from build123d import *

# Parameters (mm, degrees)
ESQUISSE2_R          = 3.75
BOSS_EXTRU_1_DEPTH   = 4
BOSS_EXTRU_1_2_DEPTH = 4
BOSS_EXTRU_1_3_DEPTH = 4
BOSS_EXTRU_1_4_DEPTH = 4
ESQUISSE3_R          = 17
ESQUISSE3_R_2        = 14.5
BOSS_EXTRU_2_DEPTH   = 4
CONG_1_R             = 2
CONG_2_R             = 2
PER_AGE1_D           = 4
PER_AGE1_DEPTH       = 93.98


with BuildPart() as part:
    # Esquisse2 → Boss.-Extru.1 (new body)
    with BuildSketch(Plane.XY):
        with Locations((-12, 12)):
            Circle(ESQUISSE2_R)
    extrude(amount=BOSS_EXTRU_1_DEPTH)



with BuildPart() as body_2:
    # Esquisse2 → Boss.-Extru.1 2 (new body)
    with BuildSketch(Plane.XY):
        with Locations((12, 12)):
            Circle(ESQUISSE2_R)
    extrude(amount=BOSS_EXTRU_1_2_DEPTH)


with BuildPart() as body_3:
    # Esquisse2 → Boss.-Extru.1 3 (new body)
    with BuildSketch(Plane.XY):
        with Locations((-12, -12)):
            Circle(ESQUISSE2_R)
    extrude(amount=BOSS_EXTRU_1_3_DEPTH)


with BuildPart() as body_4:
    # Esquisse2 → Boss.-Extru.1 4 (new body)
    with BuildSketch(Plane.XY):
        with Locations((12, -12)):
            Circle(ESQUISSE2_R)
    extrude(amount=BOSS_EXTRU_1_4_DEPTH)


with BuildPart() as part_1:
    add(part.part)

    add(body_2.part)  # Boss.-Extru.2 merges body 2

    add(body_3.part)  # Boss.-Extru.2 merges body 3

    add(body_4.part)  # Boss.-Extru.2 merges body 4
    # Esquisse3 → Boss.-Extru.2 (add)
    with BuildSketch(Plane.XY):
        Circle(ESQUISSE3_R)
        Circle(ESQUISSE3_R_2, mode=Mode.SUBTRACT)
    extrude(amount=BOSS_EXTRU_2_DEPTH)

    # Congé1
    cong_1_edges = [part_1.edges().sort_by_distance(p)[0] for p in [
        (-14.365513596, 9.09021557, 2),
        (-9.09021557, 14.365513596, 2),
        (14.365513596, 9.09021557, 2),
        (9.09021557, 14.365513596, 2),
        (-14.365513596, -9.09021557, 2),
        (-9.09021557, -14.365513596, 2),
        (9.09021557, -14.365513596, 2),
        (14.365513596, -9.09021557, 2),
    ]]
    fillet(cong_1_edges, radius=CONG_1_R)

    # Congé2
    cong_2_edges = [part_1.edges().sort_by_distance(p)[0] for p in [
        (-11.92370292, 8.250776246, 2),
        (-8.250776246, 11.92370292, 2),
        (8.250776246, 11.92370292, 2),
        (11.92370292, 8.250776246, 2),
        (-11.92370292, -8.250776246, 2),
        (-8.250776246, -11.92370292, 2),
        (8.250776246, -11.92370292, 2),
        (11.92370292, -8.250776246, 2),
    ]]
    fillet(cong_2_edges, radius=CONG_2_R)

    # Perçage1
    with Locations(Plane(origin=(0, 0, 0), x_dir=(-1, 0, 0), z_dir=(0, 0, -1))):
        with Locations((-12, 12), (12, 12), (12, -12), (-12, -12)):
            Hole(PER_AGE1_D / 2, depth=PER_AGE1_DEPTH)


solid = part_1.part
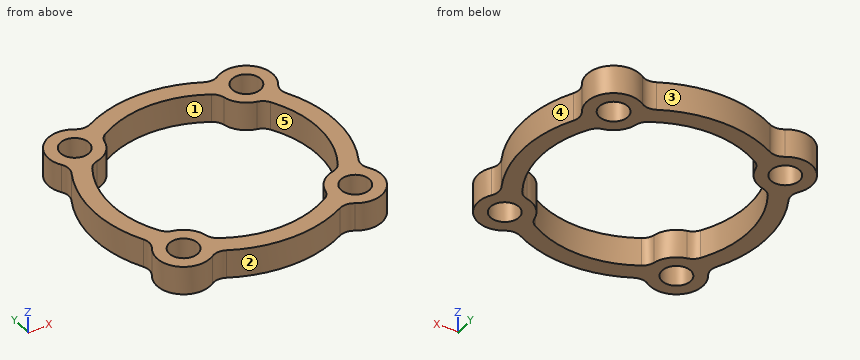
Design review of the part built by this model. Coordinates are the model's own, in mm. Face numbers are marked on the shaded views. A direction names the side the tool comes from. Give positions to 0.01 mm unless a question says otherwise; leave off trailing zeros. Loops run counter-clockwise (first coordinate to the right, second up) from the corner with the lowest first, then second, coordinate; pieces in that order, holes last. Notation, with made-up numbers: M 5.5,-19.5 L 52.5,-19.5 A27 cw 52.5,-3.5 Z; hole C 0.5,35 d10. An arc over 180 degrees is marked long. Answer as a JSON object with one key per item and string values.
Item 1: We need section B-B (z = 0.55). Count the separate pieces of the cut face and the enclosed holes in it, and give its area (3 significant figures).
Output values:
{"separate pieces": "1", "enclosed holes": "5", "area": "310 mm2"}
Item 2: Wall thickness on line 1 along Y through (x, z) = (-12, 2.95); line 2 along X through (y, z) = (-11, 0.95); line 3 along X through (y, z) = (-13, 3.45): over which ranges is each line inside the solid? List them lowest first.
Output values:
{"line 1": "y = -15.75 to -14, -10 to -7.95, 7.95 to 10, 14 to 15.75", "line 2": "x = -15.61 to -13.73, -10.27 to -8.39, 8.39 to 10.27, 13.73 to 15.61", "line 3": "x = -15.61 to -13.73, -10.27 to -6.42, 6.42 to 10.27, 13.73 to 15.61"}
Item 3: Mouldability with a two-part tool opening along Y and no side actions: class the marked faces 1, 2 and 3 as pulls with the +Y half, pulls with the -Y half, needs draft (parallel to the pull), parting line crosses it, or undercut.
Output values:
{"face 1": "undercut", "face 2": "pulls with the -Y half", "face 3": "pulls with the +Y half"}
Item 4: For P1, Ø1, axis at x = -0.5, z = 0.5, coming from the +Y side; P2, Ø8, axis at x = 4, y = 7.5, coming from the +Z side; P3, Ø2, axis at x = 7, z = 2.5, coming from the +Y side; P4, Ø2, axis at y = -3, z = 2, coming from the -X side, all flat-tipped, find the tip position at first contact; note any pin that passes through.
Output values:
{"P1": "stops at y = 17", "P2": "passes through", "P3": "stops at y = 15.91", "P4": "stops at x = -16.88"}
Item 5: Machinability: for the marked faces 4 and 5, which of the approach directions +Z, -Z, +X, -X, +Y, -Y give a long, thin tool a straight path to every point of the face, cutting with its end or side? Answer none if there is none.
Output values:
{"face 4": "+Z, -Z, +X", "face 5": "+Z, -Z"}
Item 6: We need section A-A (y = -0.5). State the section outline as (x, z) points, and give its area (3 significant figures).
Output values:
{"outline": "M -16.99,0 L -14.49,0 L -14.49,4 L -16.99,4 Z; M 14.49,0 L 16.99,0 L 16.99,4 L 14.49,4 Z", "area": "20.0 mm2"}
